Verification items for the finished model (mm, model axes). Face numbers are marked on the shaded views. A direction names the side the tool comes from. Round coordinates to 2 decimals unless told otherwise and drop trailing zeros. Write each loop counter-clockwise with the first axis right and the second up, starting at its lowest first coordinate (ties: lowest second). Pieces come first, ordered by that corner, then holes. Notation, with made-up numbers: M 22.25,-31 L 58.25,-31 A28 cw 58.25,-9 Z; hole C 10,20 d11. An arc over 180 degrees is marked long. One line per item, written item: value. Start each with the question number.
Item 1: Gauge pin test, flat ends, axial feed: pin 1 (5 mm diameter, centred on x = -12, y = -7, fed in from +Z); pin 2 (0.8 mm diameter, centred on x = -28, y = -2, fed in from -Z). Record the tip position at first contact, or that the pin passes through.
Item 2: Section check D-D, the plane z = 0.8. Record the cut outline in (x, y).
Item 3: Tool access check on the marked faces 1 and 2. Record the directions out of +Z, -Z, +X, -X, +Y, -Y that give a thin tool (end or side, any length) a straight path to the whole face; none if there is none.
Item 4: Section check C-C, the plane x = 13. Record the cut outline in (y, z).
Item 5: Draft check along X on the marked faces 3 and 4. Enter one of: +X half, -X half, draft (parallel to the pull), parting line (faces both ways), or undercut.
Item 6: Section check A-A, the plane x = -28.4. Record the cut outline in (y, z).
Item 7: Section check B-B, the plane y = -5. Record the cut outline in (x, z).
Item 8: Thickness scan on probe 1 along X at (y, z) = (1.75, 0.8); probe 2 along Y at (x, z) = (-28.4, 1.8); probe 3 along Y at (x, z) = (31.6, 2.05). Record the ranges inside material, lowest first. Write a range as from..to.
from build123d import *

# Parameters (mm, degrees)
SKETCH2_W           = 52.2
SKETCH2_H           = 21
SKETCH2_W_2         = 2.74
SKETCH2_H_2         = 10.36
BOSS_EXTRUDE1_DEPTH = 4
SKETCH2_3_W         = 2.74
SKETCH2_3_H         = 10.36
CUT_EXTRUDE1_DEPTH  = 3


with BuildPart() as part:
    # Sketch2 → Boss-Extrude1 (new body)
    # profile 1 of 3: a face of its own
    with BuildSketch(Plane.XY):
        with BuildLine():
            Line((34.6, 12.6), (34.6, -12.6))
            ThreePointArc((34.6, -12.6), (34.307106781, -13.307106781), (33.6, -13.6))
            Line((33.6, -13.6), (-30.4, -13.6))
            ThreePointArc((-30.4, -13.6), (-31.107106781, -13.307106781), (-31.4, -12.6))
            Line((-31.4, -12.6), (-31.4, 12.6))
            ThreePointArc((-31.4, 12.6), (-31.107106781, 13.307106781), (-30.4, 13.6))
            Line((-30.4, 13.6), (33.6, 13.6))
            ThreePointArc((33.6, 13.6), (34.307106781, 13.307106781), (34.6, 12.6))
        make_face()
        with BuildLine():
            ThreePointArc((-26.951988773, 9.958947861), (-27.608947861, 12.198011227), (-29.848011227, 11.541052139))
            ThreePointArc((-29.848011227, 11.541052139), (-29.191052139, 9.301988773), (-26.951988773, 9.958947861))
        make_face(mode=Mode.SUBTRACT)
        with BuildLine():
            ThreePointArc((-26.951988773, -11.541052139), (-27.608947861, -9.301988773), (-29.848011227, -9.958947861))
            ThreePointArc((-29.848011227, -9.958947861), (-29.191052139, -12.198011227), (-26.951988773, -11.541052139))
        make_face(mode=Mode.SUBTRACT)
        with BuildLine():
            ThreePointArc((33.048011227, -11.541052139), (32.391052139, -9.301988773), (30.151988773, -9.958947861))
            ThreePointArc((30.151988773, -9.958947861), (30.808947861, -12.198011227), (33.048011227, -11.541052139))
        make_face(mode=Mode.SUBTRACT)
        with BuildLine():
            ThreePointArc((33.048011227, 9.958947861), (32.391052139, 12.198011227), (30.151988773, 11.541052139))
            ThreePointArc((30.151988773, 11.541052139), (30.808947861, 9.301988773), (33.048011227, 9.958947861))
        make_face(mode=Mode.SUBTRACT)
        Rectangle(SKETCH2_W, SKETCH2_H, mode=Mode.SUBTRACT)
    # profile 2 of 3: a face of its own
    with BuildSketch(Plane.XY):
        with Locations((-28.4, -0.51)):
            Rectangle(SKETCH2_W_2, SKETCH2_H_2)
    # profile 3 of 3: a face of its own
    with BuildSketch(Plane.XY):
        with Locations((28.4, -0.51)):
            Rectangle(SKETCH2_W_2, SKETCH2_H_2)
    extrude(amount=BOSS_EXTRUDE1_DEPTH)

    # Sketch2<3> → Cut-Extrude1 (cut)
    with BuildSketch(Plane.XY):
        with Locations((-28.4, -0.51)):
            Rectangle(SKETCH2_3_W, SKETCH2_3_H)
        with Locations((28.4, -0.51)):
            Rectangle(SKETCH2_3_W, SKETCH2_3_H)
    extrude(amount=CUT_EXTRUDE1_DEPTH, mode=Mode.SUBTRACT)


solid = part.part
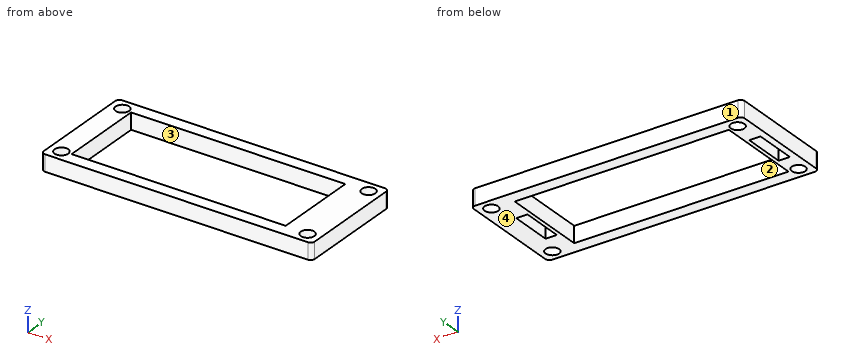
Response values:
1. pin 1: passes through
1. pin 2: stops at z = 3
2. outline: M -31.4,-12.6 A1 ccw -30.4,-13.6 L 33.6,-13.6 A1 ccw 34.6,-12.6 L 34.6,12.6 A1 ccw 33.6,13.6 L -30.4,13.6 A1 ccw -31.4,12.6 Z; hole C -28.4,-10.75 d3.3; hole C -28.4,10.75 d3.3; hole M -29.77,-5.69 L -27.03,-5.69 L -27.03,4.67 L -29.77,4.67 Z; hole M -26.1,-10.5 L 26.1,-10.5 L 26.1,10.5 L -26.1,10.5 Z; hole M 27.03,-5.69 L 29.77,-5.69 L 29.77,4.67 L 27.03,4.67 Z; hole C 31.6,-10.75 d3.3; hole C 31.6,10.75 d3.3
3. face 1: +Z, -Z, +X, -X, +Y
3. face 2: +Z, -Z
4. outline: M -13.6,0 L -10.5,0 L -10.5,4 L -13.6,4 Z; M 10.5,0 L 13.6,0 L 13.6,4 L 10.5,4 Z
5. face 3: undercut
5. face 4: draft
6. outline: M -13.6,0 L -12.4,0 L -12.4,4 L -13.6,4 Z; M -9.1,0 L -5.69,0 L -5.69,3 L 4.67,3 L 4.67,0 L 9.1,0 L 9.1,4 L -9.1,4 Z; M 12.4,0 L 13.6,0 L 13.6,4 L 12.4,4 Z
7. outline: M -31.4,0 L -29.77,0 L -29.77,3 L -27.03,3 L -27.03,0 L -26.1,0 L -26.1,4 L -31.4,4 Z; M 26.1,0 L 27.03,0 L 27.03,3 L 29.77,3 L 29.77,0 L 34.6,0 L 34.6,4 L 26.1,4 Z
8. probe 1: x = -31.4..-29.77, -27.03..-26.1, 26.1..27.03, 29.77..34.6
8. probe 2: y = -13.6..-12.4, -9.1..-5.69, 4.67..9.1, 12.4..13.6
8. probe 3: y = -13.6..-12.4, -9.1..9.1, 12.4..13.6
